Here's how the part is built. I have some questions about the finished solid (model axes, mm). A direction names the side the tool comes from. Give positions to 0.01 mm unless a question says otherwise; leave off trailing zeros. Write each loop counter-clockwise with the first axis right and the second up, starting at its lowest first coordinate (ties: lowest second). Pieces come first, ordered by that corner, then holes. Notation, with made-up numbers: (57, -19.75) - (72, -19.75) arc R26 ccw to (72, 9.25) - close; hole circle Ø8 at (64, -13). An arc over 180 degrees is marked (long way). Write each question's results on one line, items separated by ' | '. Start each with the question number.
Item 1: Please list where these lines run through material, in increasing order: line 1 along Y through (x, z) = (-452.5, 13.75); line 2 along Y through (x, z) = (-466.5, 3.25).
Item 2: Which directions (+Z, -Z, +X, -X, +Y, -Y) give clear straight access to the entire face, cutting with the end or side of a thin tool? Please do faces 1 (the flat face through (-431, 29, 2)), 2 (the flat face through (-430, 29, 0)).
Item 3: Suppose I cut it at D-D on x = -379. List the corners of the cut face in (y, z) for me.
Item 4: Suppose I cut it at A-A on x = -423. List the corners of the cut face in (y, z) for me.
Item 5: Suppose I cut it at B-B on y = 23. List the corners of the cut face in (x, z) for me, then the cut area to 3 significant figures.
Item 6: Suppose I cut it at C-C on z = 15. List the corners of the cut face in (x, y) for me.
Item 7: Will these pins go through, and if not, where does the flat tip stop? P1, Ø8, axis at y = 17, z = 8, coming from the -X side; P2, Ø14.5, axis at x = -406, y = 28.5, coming from the +Z side; P3, Ø12, axis at x = -407, z = 12, coming from the +Y side.
Autodesk Inventor part; units mm, degrees
ref_plane "YZ Plane" through (0, 0, 0) normal (1, 0, 0) x (0, 1, 0)
ref_plane "XZ Plane" through (0, 0, 0) normal (0, 1, 0) x (-1, 0, 0)
ref_plane "XY Plane" through (0, 0, 0) normal (0, 0, 1) x (1, 0, 0)
sketch "Sketch1" plane through (0, 0, 0) normal (0, 0, 1) x (1, 0, 0)
  line L0 (-490, 53) -> (490, 53)
  line L1 (490, 53) -> (490, 0)
  line L2 (490, 0) -> (-490, 0)
  line L3 (-490, 0) -> (-490, 53)
  point P0 (0, 0)
  point P1 (0, 0)
  dimension "d0" = 980
  dimension "d1" = 53
extrude "Plate1" add sketch "Sketch1" along normal blind 2
sketch "Sketch2" plane through (490, 2, 0) normal (0, -1, 0) x (1, 0, 0)
  line L0 (-980, 0) -> (0, 0)
  line L1 (0, 0) -> (0, 20)
  line L2 (0, 20) -> (-980, 20)
  line L3 (-980, 20) -> (-980, 0)
edge flange "Flange1" height 20 angle 90 thickness 2 bend radius 2.75 thickness toward (0, -1, 0) relief round relief width 2 relief depth 1 edges at (0, 0, 2) wall of the first edge with corners at (-490, 2, 0) (490, 2, 0) (490, 2, 20) (-490, 2, 20)
bend "Bend1"
corner "Corner1"
sketch "Sketch5" plane through (0, 0, 0) normal (0, 0, -1) x (-1, 0, 0)
  line L0 (490, 53) -> (-490, 53)
  line L1 (490, 0) -> (-490, 0)
  circle A0 centre (0, 53) radius 25
  line L2 (243.95, 53) -> (246.05, 53)
  line L3 (246.05, 53) -> (246.05, 27)
  line L4 (246.05, 27) -> (243.95, 27)
  line L5 (243.95, 27) -> (243.95, 53)
  line L6 (-243.95, 53) -> (-246.05, 53)
  line L7 (-246.05, 53) -> (-246.05, 27)
  line L8 (-246.05, 27) -> (-243.95, 27)
  line L9 (-243.95, 27) -> (-243.95, 53)
  line L10 (0, 53) -> (0, 0) construction
  circle A1 centre (490, 53) radius 25
  point P0 (0, 0)
  point P1 (245, 27)
  point P2 (-245, 27)
  point P3 (246.05, 53)
  point P4 (-25, 53)
  point P5 (25, 53)
  point P6 (-246.05, 53)
  dimension "d45" = 50
  dimension "d48" = 2.1
  dimension "d49" = 490
  dimension "d51" = 27
  dimension "d52" = 26
extrude "Extrusion1" cut sketch "Sketch5" against normal through all contours L3 L4 L5 L0 | L9 L8 L7 L0 | A1
sketch "Sketch9" plane through (0, 0, 2) normal (0, 0, 1) x (1, 0, 0)
  line L0 (-389.1031, 29.596) -> (-389.1031, 17.596) construction
  line L1 (-389.1031, 17.596) -> (-589.1031, 17.596) construction
  line L2 (-589.1031, 17.596) -> (-589.1031, 29.596) construction
  line L3 (-589.1031, 29.596) -> (-389.1031, 29.596) construction
  line L4 (-490, 53) -> (490, 53)
  point P0 (0, 0)
  point P1 (1.05, 68)
  point P2 (490, 53)
  point P3 (-490, 53)
  dimension "d40" = 200
  dimension "d41" = 12
mark "Mark2"
sketch "Sketch10" plane through (-490, 0, 20) normal (0, -1, 0) x (1, 0, 0)
  line L0 (980, -20) -> (736.05, -20)
  line L1 (0, 0) -> (980, 0)
  line L2 (980, -20) -> (97.2902, -20)
  line L3 (97.2902, -20) -> (97.2902, 0)
  line L4 (97.2902, 0) -> (980, 0)
  line L5 (980, 0) -> (980, -20)
  line L6 (97.2902, 0) -> (121.1253, -20)
  point P0 (490, -20)
  point P1 (736.05, -20)
  dimension "d53" = 882.7098
  dimension "d54" = 50
extrude "Extrusion4" cut sketch "Sketch10" against normal through all contours L0 L2 L6 L1 L5
equation "\"d2\" = Thickness"
equation "\"d3\" = BendReliefWidth"
equation "\"d4\" = BendReliefDepth"
equation "\"d5\" = MinimumRemnant"
equation "\"d6\" = TransitionRadius"
equation "\"d9\" = BendRadius"
equation "\"d10\" = CornerReliefSize"
equation "\"d11\" = GapSize"
equation "\"d12\" = JacobiRadiusSize"
equation "\"BendReliefWidth\" = Thickness"
equation "\"BendReliefDepth\" = 0.5 * Thickness"
equation "\"CornerReliefSize\" = 4 * Thickness"
equation "\"MinimumRemnant\" = 2 * Thickness"
equation "\"TransitionRadius\" = BendRadius"
equation "\"JacobiRadiusSize\" = BendRadius"
equation "\"GapSize\" = Thickness"
properties part number "MSC 330 STRINGER BOARD  ###" material "Stainless Steel"
Checked values:
1) line 1: y = 0 to 2 | line 2: y = 0.24 to 2.45
2) face 1: +Z, +X, -X, +Y | face 2: -Z, +X, -X, +Y, -Y
3) outline: (0, 4.75) arc R4.75 ccw to (4.75, 0) - (53, 0) - (53, 2) - (4.75, 2) arc R2.75 cw to (2, 4.75) - (2, 8.5) - (0, 8.5) - close
4) outline: (0, 4.75) arc R4.75 ccw to (4.75, 0) - (53, 0) - (53, 2) - (4.75, 2) arc R2.75 cw to (2, 4.75) - (2, 20) - (0, 20) - close
5) outline: (-490, 0) - (-368.87, 0) - (-371.26, 2) - (-490, 2) - close | area: 240 mm^2
6) outline: (-490, 0) - (-386.75, 0) - (-386.75, 2) - (-490, 2) - close
7) P1: passes through | P2: stops at z = 2 | P3: stops at y = 2
